The model under review builds one solid part; all positions refer to its coordinate system, in mm. Give positions to 0.01 mm unless a question says otherwise; leave off trailing zeros. Loops run counter-clockwise (first coordinate to the right, second up) from the corner with the lowest first, then second, coordinate; pieces in that order, holes last. Notation, with made-up numbers: (11, 4.5) - (26, 4.5) arc R32 ccw to (26, 40.5) - close; hole circle Ø5 at (65, -0.75). An arc over 180 degrees is marked (long way). Return JSON: item names as keys, results as strings. Group by question number.
Autodesk Inventor part; units mm, degrees
ref_plane "Work Plane3" through (0, 9.525, 0) normal (0, 0.7071, 0.7071) x (-1, 0, 0)
ref_plane "YZ Plane" through (0, 0, 0) normal (1, 0, 0) x (0, 1, 0)
ref_plane "XY Plane" through (0, 0, 0) normal (0, 0, 1) x (1, 0, 0)
sketch "Sketch1" plane through (0, 0, 0) normal (0, 0, 1) x (1, 0, 0)
  circle A0 centre (0, 0) radius 9.525
  dimension "d0" = 19.05
extrude "Extrusion1" add sketch "Sketch1" along normal blind 36.576
ref_plane "Work Plane2" through (0, 15.875, 0) normal (0, 1, 0) x (-1, 0, 0)
sketch "Sketch4" plane through (0, 15.875, 0) normal (0, 1, 0) x (-1, 0, 0)
  circle A0 centre (0, 7.62) radius 1.4605
  point P0 (0, 0)
  dimension "d6" = 2.921
  dimension "d7" = 7.62
sketch "Sketch5" plane through (0, 0, 0) normal (0, 0, -1) x (-1, 0, 0)
  circle A0 centre (0, 0) radius 9.525
  circle A1 centre (0, 1.905) radius 1.4605
  line L0 (0, 9.525) -> (14.2875, 9.525)
  dimension "d8" = 2.921
  dimension "d9" = 7.62
ref_plane "Work Plane3" through (0, 9.525, 0) normal (0, 0.7071, 0.7071) x (-1, 0, 0)
sketch "Sketch6" plane through (0, 9.525, 0) normal (0, 0.7071, 0.7071) x (-1, 0, 0)
  circle A0 centre (0, 3.9683) radius 1.5875
  point P0 (0, 6.7352)
  dimension "d11" = 3.175
extrude "Extrusion2" add sketch "Sketch6" along normal mid plane 25.4
sketch "Sketch7" plane through (0, -2.2613, -6.1742) normal (0, -0.7071, -0.7071) x (-1, 0, 0)
  circle A0 centre (0, 0) radius 1.5875
  circle A1 centre (0, 0) radius 1.5875
  point P0 (0, -2.7669)
hole "Hole1" at (-0.0004, -2.2603, -6.1752) direction (0, 0.7071, 0.7071) diameter 3.302 depth 25.4 tip angle 118
properties part number "Stainless Steel"
1) We need section B-B, the plane x = 6.5. Write out the cut boundary in (y, z).
2) We need section A-A, the plane z = 16. Write out the cut boundary in (x, y) (3 decimals), plus the area to 3 significant figures.
3) For pin 1 Ø2 at (x, z) = (2.5, 26) entering from -Y; pin 2 Ø6 at (x, z) = (-4, 20.5) entering from +Y; pin 3 Ø6 at (y, z) = (-4.5, 27) entering from +X, all flat-tipped, find the tip position at first contact; note any pin that passes through.
4) Draft analysis for pull direction X (two halves, no side actions). For faces 1 (the face through (0, 0, 0)), 2 (the face through (-0.07, 5.6, 4.02)), 3 (the face through (-7.559, 5.796, 18.032)), state which applies: +X half, -X half, draft (parallel to the pull), parting line (faces both ways), or undercut.
5) To check wall thickness, follow line 1 (X direction, y = 6.25, z = 3.5); line 2 (X direction, y = 7.75, z = 33.5); line 3 (Y direction, x = -3.75, z = 6). State the ranges of each line that lie inside material, in increasing order.
Findings:
{
 "1": {"outline": "(-6.96, 0) - (6.96, 0) - (6.96, 36.58) - (-6.96, 36.58) - close"},
 "2": {"outline": "circle Ø19.05 at (0, 0)", "area": "285 mm^2"},
 "3": {"pin 1": "stops at y = -9.41", "pin 2": "stops at y = 9.47", "pin 3": "stops at x = 9.41"},
 "4": {"face 1": "draft", "face 2": "undercut", "face 3": "parting line"},
 "5": {"line 1": "x = -7.19 to -1.43, 1.43 to 7.19", "line 2": "x = -5.54 to 5.54", "line 3": "y = -8.76 to 8.76"}
}
